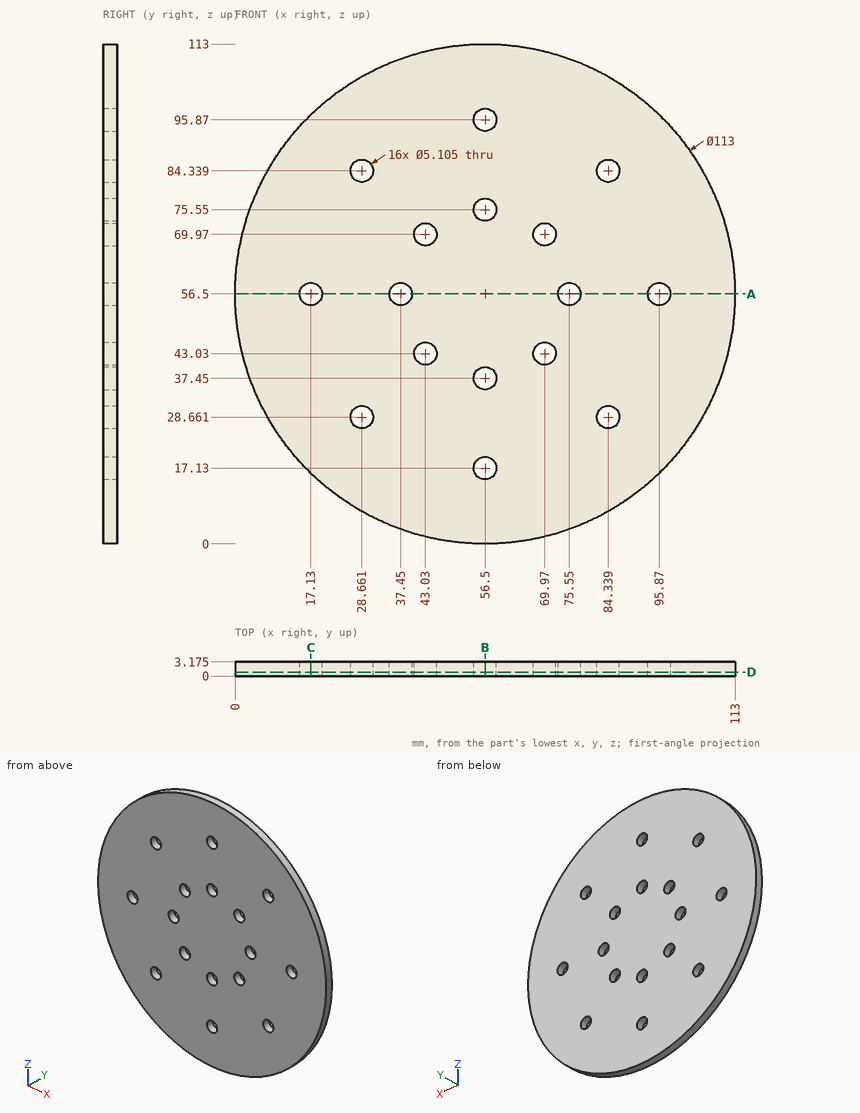
Could you check a few things on this drawing? It's one solid part, dimensions in mm from its lowest x, y, z. Give positions to 0.01 mm unless a question says otherwise; leave off trailing zeros. Order: outer loops, then holes, each group sorted by start corner. A loop starts at its lowest first (then second) coordinate and runs counter-clockwise, first axis right, second up. Notation, with made-up numbers: (22, 73) -> (81, 73) arc R32 ccw to (81, 102) -> close; hole circle Ø1 at (53, 65.25). An arc over 180 degrees is marked (long way). Answer in a Markdown table with one row per item. Add a question column.
Item 1: I'm going to push flat-ended pins straight in: P1, Ø1, axis at y = 1, z = 64, coming from the +X side (1 decimal); P2, Ø3, axis at x = 56.5, z = 37.45, coming from the -Y side; P3, Ø1.5, axis at y = 2, z = 14.5, coming from the +X side. Where does each tip first touch, or does it pass through?
Item 2: Imagine slicing it at C-C (x = 17.13). List the corners of the cut face in (y, z) for me (1 decimal), and give its area (3 significant figures).
Item 3: Imagine slicing it at D-D (y = 0.85). Count the separate pieces of the cut face and the enclosed holes in it, and give its area (3 significant figures).
Item 4: Please list where these lines run through material, in increasing order: probe 1 along X at (y, z) = (1.65, 56.5); probe 2 along Z at (x, y) = (55, 1.7) (1 decimal); probe 3 along X at (y, z) = (1.6, 43).
Item 5: Imagine slicing it at B-B (x = 56.5). List the corners of the cut face in (y, z) for me (1 decimal).
Item 6: Imagine slicing it at A-A (z = 56.5). List the corners of the cut face in (x, y) for me (1 decimal), and give its area (3 significant figures).
Result:
| question | item | result |
|---|---|---|
| 1 | P1 | x = 112.6 |
| 1 | P2 | through |
| 1 | P3 | x = 95.11 |
| 2 | outline | (0, 16) -> (3.2, 16) -> (3.2, 53.9) -> (0, 53.9) -> close; (0, 59.1) -> (3.2, 59.1) -> (3.2, 97) -> (0, 97) -> close |
| 2 | area | 241 mm2 |
| 3 | separate pieces | 1 |
| 3 | enclosed holes | 16 |
| 3 | area | 9,700 mm2 |
| 4 | probe 1 | 0 to 14.58, 19.68 to 34.9, 40 to 73, 78.1 to 93.32, 98.42 to 113 |
| 4 | probe 2 | 0 to 15.1, 19.2 to 35.4, 39.5 to 73.5, 77.6 to 93.8, 97.9 to 113 |
| 4 | probe 3 | 1.64 to 40.48, 45.58 to 67.42, 72.52 to 111.36 |
| 5 | outline | (0, 0) -> (3.2, 0) -> (3.2, 14.6) -> (0, 14.6) -> close; (0, 19.7) -> (3.2, 19.7) -> (3.2, 34.9) -> (0, 34.9) -> close; (0, 40) -> (3.2, 40) -> (3.2, 73) -> (0, 73) -> close; (0, 78.1) -> (3.2, 78.1) -> (3.2, 93.3) -> (0, 93.3) -> close; (0, 98.4) -> (3.2, 98.4) -> (3.2, 113) -> (0, 113) -> close |
| 6 | outline | (0, 0) -> (14.6, 0) -> (14.6, 3.2) -> (0, 3.2) -> close; (19.7, 0) -> (34.9, 0) -> (34.9, 3.2) -> (19.7, 3.2) -> close; (40, 0) -> (73, 0) -> (73, 3.2) -> (40, 3.2) -> close; (78.1, 0) -> (93.3, 0) -> (93.3, 3.2) -> (78.1, 3.2) -> close; (98.4, 0) -> (113, 0) -> (113, 3.2) -> (98.4, 3.2) -> close |
| 6 | area | 294 mm2 |
